Geometry: see drawing. Coordinates: mm, zero at the bounding-box minimum. Coordinates: 2 decimals unless noted, no trailing zeros. Loops run counter-clockwise (first coordinate to the right, second up) from the corner with the lowest first, then second, coordinate; pieces in that order, holes last.
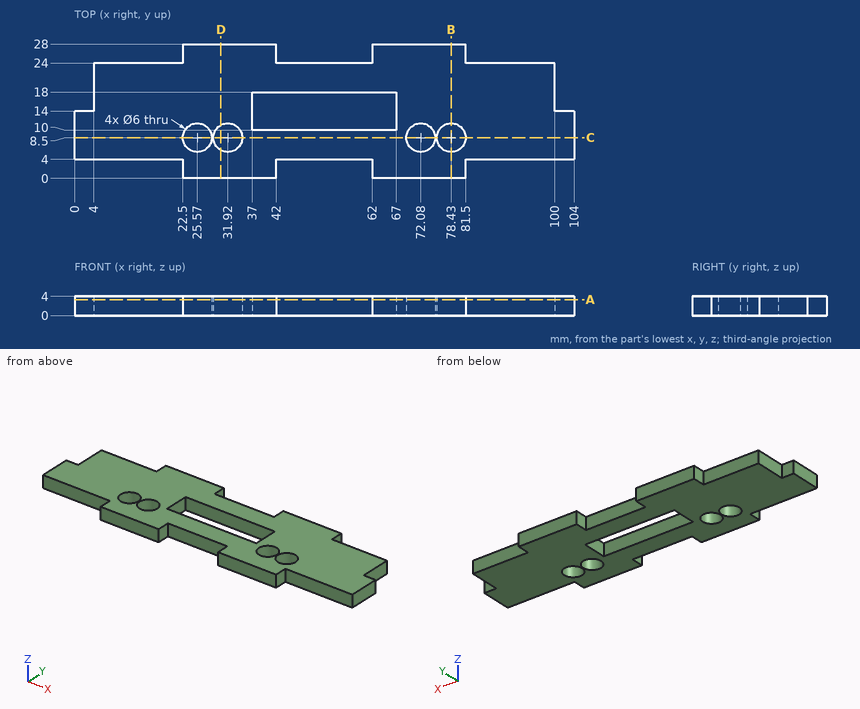
Item 1: Contact query for flat-ended pins moving along their axis: P1, Ø1.2, axis at x = 91.5, z = 2.5, coming from the +Y side; P2, Ø2, axis at y = 1.5, z = 3, coming from the +X side; P3, Ø2, axis at x = 89.5, z = 1.5, coming from the -Y side. Output: stop coordinate, or through.
Result:
P1: stops at y = 24
P2: stops at x = 81.5
P3: stops at y = 4
Item 2: Section query C-C (y = 8.5). Output: boundary loops of the cut face in (x, z).
Result:
outline: (0, 0) - (22.57, 0) - (22.57, 4) - (0, 4) - close; (28.57, 0) - (28.92, 0) - (28.92, 4) - (28.57, 4) - close; (34.92, 0) - (69.08, 0) - (69.08, 4) - (34.92, 4) - close; (75.08, 0) - (75.43, 0) - (75.43, 4) - (75.08, 4) - close; (81.43, 0) - (104, 0) - (104, 4) - (81.43, 4) - close
Item 3: Section query A-A (z = 3.35). Count the separate pieces of the cut face and the enclosed holes in it, then the cut area to 3 significant figures.
Result:
separate pieces: 1
enclosed holes: 5
area: 1,960 mm2
Item 4: Section query D-D (x = 30.5). Output: boundary loops of the cut face in (y, z), then the cut area to 3 significant figures.
Result:
outline: (0, 0) - (5.86, 0) - (5.86, 4) - (0, 4) - close; (11.14, 0) - (28, 0) - (28, 4) - (11.14, 4) - close
area: 90.9 mm2
Item 5: Line query: L1, parallel to X at y = 8.5, z = 0.85; L2, parallel to Y at x = 55, z = 3; L3, parallel to Y at x = 31.92, z = 1.2. Output: solid intervals per line, ascending.
Result:
L1: x = 0 to 22.57, 28.57 to 28.92, 34.92 to 69.08, 75.08 to 75.43, 81.43 to 104
L2: y = 4 to 10, 18 to 24
L3: y = 0 to 5.5, 11.5 to 28
Item 6: Section query B-B (x = 78.43). Output: boundary loops of the cut face in (y, z).
Result:
outline: (0, 0) - (5.5, 0) - (5.5, 4) - (0, 4) - close; (11.5, 0) - (28, 0) - (28, 4) - (11.5, 4) - close
